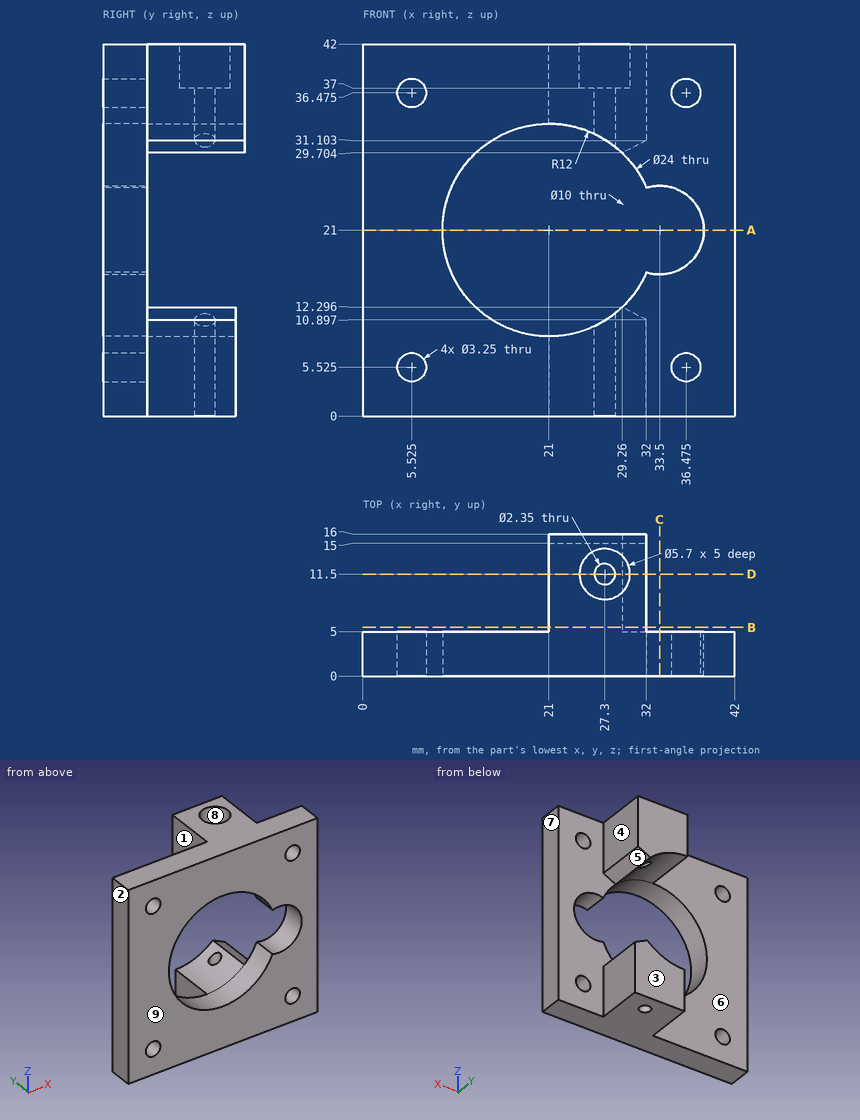
Could you check a few things on this drawing? It's one solid part, dimensions in mm from its lowest x, y, z. A direction names the side the tool comes from. Round coordinates to 2 decimals unless told otherwise and drop trailing zeros. Order: outer loops, then holes, each group sorted by start corner. A loop starts at its lowest first (then second) coordinate and runs counter-clockwise, first axis right, second up.
Q1. I'm going to push flat-ended pins straight in: P1, Ø1, axis at x = 34, z = 30.5, coming from the +Y side; P2, Ø3, axis at x = 27.3, y = 11.5, coming from the -Z side; P3, Ø1.9, axis at x = 5.525, z = 5.525, coming from the -Y side; P4, Ø5.5, axis at x = 24, z = 4.5, coming from the +Y side. Where does each tip first touch, or does it pass through?
Geometry says:
P1: stops at y = 5
P2: stops at z = 0
P3: passes through
P4: stops at y = 15
Q2. Imagine slicing it at B-B, the plane y = 5.5. List the corners of the cut face in (x, z) for me (1 decimal), then the cut area to 3 significant figures.
Geometry says:
outline: (21, 0) - (32, 0) - (32, 10.9) - (29.3, 12.3) arc R12 cw to (21, 9) - close; (21, 33) arc R12 cw to (29.3, 29.7) - (32, 31.1) - (32, 42) - (21, 42) - close
area: 229 mm2
Q3. Imagine slicing it at C-C, the plane x = 33.5. List the corners of the cut face in (y, z) for me.
Geometry says:
outline: (0, 0) - (5, 0) - (5, 16) - (0, 16) - close; (0, 26) - (5, 26) - (5, 42) - (0, 42) - close
Q4. Imagine slicing it at A-A, the plane z = 21. List the corners of the cut face in (x, y) for me, then the cut area to 3 significant figures.
Geometry says:
outline: (0, 0) - (9, 0) - (9, 5) - (0, 5) - close; (38.5, 0) - (42, 0) - (42, 5) - (38.5, 5) - close
area: 62.5 mm2
Q5. Which directions (+Z, -Z, +X, -X, +Y, -Y) give clear straight access to the entire face, cutting with the end or side of a thin tool? Please do the marked faces 1, 2, 3, 4 and 5.
Geometry says:
face 1: +Z, -Z, -X, +Y
face 2: +Z, -Z, -X, +Y, -Y
face 3: -Z, +X, -X, +Y
face 4: +Z, -Z, +X, +Y
face 5: +X, +Y
Q6. Thinking about a two-plate mould opening in Y: for the marked faces 6, 7, 8 and 9, which applies, released by +Y, released by -Y, zero draft, split by the parting line, or undercut?
Geometry says:
face 6: released by +Y
face 7: zero draft
face 8: undercut
face 9: released by -Y
Q7. Imagine slicing it at D-D, the plane y = 11.5. State how many separate pieces and enclosed holes the cut face has, then the cut area to 3 significant figures.
Geometry says:
separate pieces: 4
enclosed holes: 0
area: 162 mm2
Q8. Please list where these lines run through material, in increasing order: probe 1 along Y at (x, z) = (27.3, 39.45); probe 2 along X at (y, z) = (11.5, 35.25) (1 decimal); probe 3 along Z at (x, y) = (6, 2.75).
Geometry says:
probe 1: y = 0 to 8.65, 14.35 to 16
probe 2: x = 21 to 26.1, 28.5 to 32
probe 3: z = 0 to 3.97, 7.08 to 34.92, 38.03 to 42
